Input: part model. Units: mm. Frame: model coordinates. A direction names the side the tool comes from. Give positions to 0.01 mm unless a question says otherwise; leave off trailing zeros. Loops run counter-clockwise (first coordinate to the right, second up) from the corner with the lowest first, then second, coordinate; pieces in that order, holes last. Notation, with made-up numbers: (67, 2.25) -> (71, 2.25) arc R23 ccw to (71, 11.25) -> close; hole circle Ø4 at (17, 15). An arc over 180 degrees is marked (long way). Answer in a Markdown table with one row per item. Add a question column.
```python
from build123d import *

# Parameters (mm, degrees)
F2_R     = 2.413
F3_DEPTH = 25.4
F4_R     = 3.175


with BuildPart() as f1:
    # F0 (on Front) → F1 (revolve)
    with BuildSketch(Plane.XZ):
        Polygon((-19.05, 0), (-3.302, 0), (-3.302, 12.7), (-9.652, 12.7), (-9.652, 6.35), (-19.05, 6.35), align=None)
    revolve(axis=Axis((0, 0, 14.768198), (0, 0, 1)))

    # F2 (on face) → F3 (cut)
    with BuildSketch(Plane(origin=(0, 0, 0), x_dir=(1, 0, 0), z_dir=(0, 0, -1))):
        with Locations((0, -14.224)):
            Circle(F2_R)
        with Locations((0, 14.224)):
            Circle(F2_R)
    extrude(amount=-F3_DEPTH, mode=Mode.SUBTRACT)

    # F4
    f4_edges = [f1.edges().sort_by_distance(p)[0] for p in [
        (9.652, 0, 12.7),
    ]]
    fillet(f4_edges, radius=F4_R)


solid = f1.part
```
1) Section C-C on z = 7.5. Output: boundary loops of the cut face in (x, y), and give its area (3 significant figures).
2) Section D-D on x = 12. Output: boundary loops of the cut face in (y, z), and give its area (3 significant figures).
3) Pull-direction query (Y, two-part tool) for faces 3 (the face through (15.12, 11.59, 3.13)), 4 (the face through (-3.05, 1.26, 6.44)), 5 (the face through (-9, -5, 6.35)); classes: +Y half, -Y half, draft (parallel to the pull), parting line (faces both ways), or undercut.
4) Section B-B on y = 0. Output: boundary loops of the cut face in (x, z) (3 decimals), and give its area (3 significant figures).
5) Section A-A on x = 0. Output: boundary loops of the cut face in (y, z) (3 decimals).
6) Pin query (flat end, axial travel): pin 1 (6 mm diameter, centred on x = 0, y = 0, fed in from +Z) (3 decimals); pin 2 (5.5 mm diameter, centred on x = 0, y = 14.224, fed in from +Z); pin 3 (12 mm diameter, centred on x = 6.5, y = -11, fed in from +Z). Return the tip coordinate at first contact, or that it passes through.
7) Material intervals for line 1 along Y through (x, z) = (0, 2.75); line 2 along X through (y, z) = (0, 8.5); line 3 along Z through (x, y) = (13, 10), sorted ascending.
8) Reachability of faces 1 (the face through (7.66, 5.87, 7.92)), 2 (the face through (-0.523, -11.868, 3.131)) from +Z, -Z, +X, -X, +Y, -Y: full face, straight path, thin tool, end or side. Return the list, or none.
Working result:
| question | item | result |
|---|---|---|
| 1 | outline | circle Ø19.3 at (0, 0); hole circle Ø6.6 at (0, 0) |
| 1 | area | 258 mm2 |
| 2 | outline | (-14.8, 0) -> (14.8, 0) -> (14.8, 6.35) -> (-14.8, 6.35) -> close |
| 2 | area | 188 mm2 |
| 3 | face 3 | parting line |
| 3 | face 4 | undercut |
| 3 | face 5 | draft |
| 4 | outline | (-19.05, 0) -> (-3.302, 0) -> (-3.302, 12.7) -> (-6.477, 12.7) arc R3.175 ccw to (-9.652, 9.525) -> (-9.652, 6.35) -> (-19.05, 6.35) -> close; (3.302, 0) -> (19.05, 0) -> (19.05, 6.35) -> (9.652, 6.35) -> (9.652, 9.525) arc R3.175 ccw to (6.477, 12.7) -> (3.302, 12.7) -> close |
| 4 | area | 276 mm2 |
| 5 | outline | (-19.05, 0) -> (-16.637, 0) -> (-16.637, 6.35) -> (-19.05, 6.35) -> close; (-11.811, 0) -> (-3.302, 0) -> (-3.302, 12.7) -> (-6.477, 12.7) arc R3.175 ccw to (-9.652, 9.525) -> (-9.652, 6.35) -> (-11.811, 6.35) -> close; (3.302, 0) -> (11.811, 0) -> (11.811, 6.35) -> (9.652, 6.35) -> (9.652, 9.525) arc R3.175 ccw to (6.477, 12.7) -> (3.302, 12.7) -> close; (16.637, 0) -> (19.05, 0) -> (19.05, 6.35) -> (16.637, 6.35) -> close |
| 6 | pin 1 | passes through |
| 6 | pin 2 | stops at z = 6.35 |
| 6 | pin 3 | stops at z = 12.69 |
| 7 | line 1 | y = -19.05 to -16.64, -11.81 to -3.3, 3.3 to 11.81, 16.64 to 19.05 |
| 7 | line 2 | x = -9.65 to -3.3, 3.3 to 9.65 |
| 7 | line 3 | z = 0 to 6.35 |
| 8 | face 1 | +Z |
| 8 | face 2 | +Z, -Z |
